Build history of the part. All positions in model axes, mm. Give positions to 0.01 mm unless a question says otherwise; leave off trailing zeros. One line per item, written item: value. Start each with the question number.
from build123d import *

# Parameters (mm, degrees)
BOSS_EXTRUDE1_DEPTH   = 1000
SKETCH3_R             = 3.4
CUT_EXTRUDE1_DEPTH    = 1000
CUT_EXTRUDE2_DEPTH    = 1000
FILLET1_R             = 1
FILLET2_R             = 1
FILLET3_R             = 1
CUT_EXTRUDE3_DEPTH    = 1000
CUT_EXTRUDE4_DEPTH    = 1000
FILLET4_R             = 1
FILLET5_R             = 1
FILLET6_R             = 1
FILLET7_R             = 1
FILLET8_R             = 1
FILLET9_R             = 1
FILLET10_R            = 1
FILLET11_R            = 1
MIRROR11_COPY_1_DEPTH = 1000
MIRROR11_COPY_2_DEPTH = 1000
CUT_EXTRUDE5_DEPTH    = 1000


with BuildPart() as part:
    # Sketch1 → Boss-Extrude1 (new body)
    with BuildSketch(Plane(origin=(0, 0, 0), x_dir=(1, 0, 0), z_dir=(0, 1, 0))):
        with BuildLine():
            Line((5, 0), (75, 0))
            ThreePointArc((75, 0), (78.535533906, -1.464466094), (80, -5))
            Line((80, -5), (80, -35))
            ThreePointArc((80, -35), (78.535533906, -38.535533906), (75, -40))
            Line((75, -40), (5, -40))
            ThreePointArc((5, -40), (1.464466094, -38.535533906), (0, -35))
            Line((0, -35), (0, -5))
            ThreePointArc((0, -5), (1.464466094, -1.464466094), (5, 0))
        make_face()
    extrude(amount=BOSS_EXTRUDE1_DEPTH)

    # Sketch3 → Cut-Extrude1 (cut)
    with BuildSketch(Plane(origin=(0, 1000, 0), x_dir=(1, 0, 0), z_dir=(0, 1, 0))):
        with Locations(Location((20, -20, 0), (0, 0, 270))):
            Circle(SKETCH3_R)
    cut_extrude1 = extrude(amount=-CUT_EXTRUDE1_DEPTH, mode=Mode.SUBTRACT)

    # Mirror3: Cut-Extrude1 across plane
    add(cut_extrude1.mirror(Plane(origin=(40, 0, 0), x_dir=(0, 0, 1), z_dir=(1, 0, 0))), mode=Mode.SUBTRACT)

    # Sketch7 → Cut-Extrude2 (cut)
    with BuildSketch(Plane(origin=(0, 0, 0), x_dir=(-1, 0, 0), z_dir=(0, -1, 0))):
        with BuildLine():
            Line((-15.9, -40), (-24.1, -40))
            Line((-24.1, -40), (-24.1, -36.5))
            ThreePointArc((-24.1, -36.5), (-24.392893219, -35.792893219), (-25.1, -35.5))
            Line((-25.1, -35.5), (-29.489753594, -35.5))
            ThreePointArc((-29.489753594, -35.5), (-30.415270825, -34.8787055), (-30.190750526, -33.786835712))
            Line((-30.190750526, -33.786835712), (-24.391814382, -28.086835712))
            ThreePointArc((-24.391814382, -28.086835712), (-24.069522951, -27.874482769), (-23.69081745, -27.8))
            Line((-23.69081745, -27.8), (-16.309186536, -27.8))
            ThreePointArc((-16.309186536, -27.8), (-15.930477876, -27.874484063), (-15.608184734, -28.086840499))
            Line((-15.608184734, -28.086840499), (-9.809327805, -33.786840499))
            ThreePointArc((-9.809327805, -33.786840499), (-9.584813669, -34.87870866), (-10.510329607, -35.5))
            Line((-10.510329607, -35.5), (-14.9, -35.5))
            ThreePointArc((-14.9, -35.5), (-15.607106781, -35.792893219), (-15.9, -36.5))
            Line((-15.9, -36.5), (-15.9, -40))
        make_face()
    cut_extrude2 = extrude(amount=-CUT_EXTRUDE2_DEPTH, mode=Mode.SUBTRACT)

    # Fillet1
    fillet1_edges = [part.edges().sort_by_distance(p)[0] for p in [
        (15.9, 500, 40),
        (24.1, 500, 40),
    ]]
    fillet(fillet1_edges, radius=FILLET1_R)

    # Mirror8: Cut-Extrude2 across plane
    add(cut_extrude2.mirror(Plane(origin=(40, 0, 0), x_dir=(0, 0, 1), z_dir=(1, 0, 0))), mode=Mode.SUBTRACT)

    # Fillet2
    fillet2_edges = [part.edges().sort_by_distance(p)[0] for p in [
        (55.9, 500, 40),
    ]]
    fillet(fillet2_edges, radius=FILLET2_R)

    # Fillet3
    fillet3_edges = [part.edges().sort_by_distance(p)[0] for p in [
        (64.1, 500, 40),
    ]]
    fillet(fillet3_edges, radius=FILLET3_R)

    # Sketch9 → Cut-Extrude3 (cut)
    with BuildSketch(Plane(origin=(0, 0, 0), x_dir=(1, 0, 0), z_dir=(0, 1, 0))):
        with BuildLine():
            Line((14.899846923, -4.500713815), (10.450461284, -4.500713815))
            ThreePointArc((10.450461284, -4.500713815), (9.526581751, -5.118030383), (9.743354502, -6.207820596))
            Line((9.743354502, -6.207820596), (15.442640687, -11.907106781))
            ThreePointArc((15.442640687, -11.907106781), (15.767064036, -12.123879533), (16.149747468, -12.2))
            Line((16.149747468, -12.2), (23.850252532, -12.2))
            ThreePointArc((23.850252532, -12.2), (24.232935964, -12.123879533), (24.557359313, -11.907106781))
            Line((24.557359313, -11.907106781), (30.257359313, -6.207106781))
            ThreePointArc((30.257359313, -6.207106781), (30.474132064, -5.117316568), (29.550252532, -4.5))
            Line((29.550252532, -4.5), (25.099846964, -4.5))
            ThreePointArc((25.099846964, -4.5), (24.392724723, -4.207091321), (24.099846965, -3.499956273))
            Line((24.099846965, -3.499956273), (24.100000008, 0))
            Line((24.100000008, 0), (15.9, 0))
            Line((15.9, 0), (15.899846922, -3.500757542))
            ThreePointArc((15.899846922, -3.500757542), (15.606938244, -4.207836056), (14.899846923, -4.500713815))
        make_face()
    cut_extrude3 = extrude(amount=CUT_EXTRUDE3_DEPTH, mode=Mode.SUBTRACT)

    # Mirror9: Cut-Extrude3 across plane
    add(cut_extrude3.mirror(Plane(origin=(40, 0, 0), x_dir=(0, 0, 1), z_dir=(1, 0, 0))), mode=Mode.SUBTRACT)

    # Sketch10 → Cut-Extrude4 (cut)
    with BuildSketch(Plane(origin=(0, 0, 0), x_dir=(1, 0, 0), z_dir=(0, 1, 0))):
        with BuildLine():
            Line((4.5, -14.9), (4.5, -10.58605332))
            ThreePointArc((4.5, -10.58605332), (5.126159695, -9.658560233), (6.220486853, -9.892584724))
            Line((6.220486853, -9.892584724), (11.920486853, -15.814662646))
            ThreePointArc((11.920486853, -15.814662646), (12.127493087, -16.134290938), (12.2, -16.508131242))
            Line((12.2, -16.508131242), (12.2, -23.491868758))
            ThreePointArc((12.2, -23.491868758), (12.127493087, -23.865709062), (11.920486853, -24.185337354))
            Line((11.920486853, -24.185337354), (6.220486853, -30.107415276))
            ThreePointArc((6.220486853, -30.107415276), (5.126159695, -30.341439767), (4.5, -29.41394668))
            Line((4.5, -29.41394668), (4.5, -25.1))
            ThreePointArc((4.5, -25.1), (4.207106781, -24.392893219), (3.5, -24.1))
            Line((3.5, -24.1), (0, -24.1))
            Line((0, -24.1), (0, -15.9))
            Line((0, -15.9), (3.5, -15.9))
            ThreePointArc((3.5, -15.9), (4.207106781, -15.607106781), (4.5, -14.9))
        make_face()
    cut_extrude4 = extrude(amount=CUT_EXTRUDE4_DEPTH, mode=Mode.SUBTRACT)

    # Fillet4
    fillet4_edges = [part.edges().sort_by_distance(p)[0] for p in [
        (24.100000008, 500, 0),
    ]]
    fillet(fillet4_edges, radius=FILLET4_R)

    # Fillet5
    fillet5_edges = [part.edges().sort_by_distance(p)[0] for p in [
        (64.1, 500, 0),
    ]]
    fillet(fillet5_edges, radius=FILLET5_R)

    # Fillet6
    fillet6_edges = [part.edges().sort_by_distance(p)[0] for p in [
        (55.899999992, 500, 0),
    ]]
    fillet(fillet6_edges, radius=FILLET6_R)

    # Fillet7
    fillet7_edges = [part.edges().sort_by_distance(p)[0] for p in [
        (15.9, 500, 0),
    ]]
    fillet(fillet7_edges, radius=FILLET7_R)

    # Fillet8
    fillet8_edges = [part.edges().sort_by_distance(p)[0] for p in [
        (0, 500, 24.1),
    ]]
    fillet(fillet8_edges, radius=FILLET8_R)

    # Fillet9
    fillet9_edges = [part.edges().sort_by_distance(p)[0] for p in [
        (0, 500, 15.9),
    ]]
    fillet(fillet9_edges, radius=FILLET9_R)

    # Mirror10: Cut-Extrude4 across plane
    add(cut_extrude4.mirror(Plane(origin=(40, 0, 0), x_dir=(0, 0, 1), z_dir=(1, 0, 0))), mode=Mode.SUBTRACT)

    # Fillet10
    fillet10_edges = [part.edges().sort_by_distance(p)[0] for p in [
        (80, 500, 15.9),
    ]]
    fillet(fillet10_edges, radius=FILLET10_R)

    # Fillet11
    fillet11_edges = [part.edges().sort_by_distance(p)[0] for p in [
        (80, 500, 24.1),
    ]]
    fillet(fillet11_edges, radius=FILLET11_R)

    # Mirror11 copy 1 sketch → Mirror11 copy 1 (cut)
    with BuildSketch(Plane(origin=(40, 0, 0), x_dir=(1, 0, 0), z_dir=(0, 1, 0))):
        with BuildLine():
            Line((4.5, -14.9), (4.5, -10.58605332))
            ThreePointArc((4.5, -10.58605332), (5.126159695, -9.658560233), (6.220486853, -9.892584724))
            Line((6.220486853, -9.892584724), (11.920486853, -15.814662646))
            ThreePointArc((11.920486853, -15.814662646), (12.127493087, -16.134290938), (12.2, -16.508131242))
            Line((12.2, -16.508131242), (12.2, -23.491868758))
            ThreePointArc((12.2, -23.491868758), (12.127493087, -23.865709062), (11.920486853, -24.185337354))
            Line((11.920486853, -24.185337354), (6.220486853, -30.107415276))
            ThreePointArc((6.220486853, -30.107415276), (5.126159695, -30.341439767), (4.5, -29.41394668))
            Line((4.5, -29.41394668), (4.5, -25.1))
            ThreePointArc((4.5, -25.1), (4.207106781, -24.392893219), (3.5, -24.1))
            Line((3.5, -24.1), (0, -24.1))
            Line((0, -24.1), (0, -15.9))
            Line((0, -15.9), (3.5, -15.9))
            ThreePointArc((3.5, -15.9), (4.207106781, -15.607106781), (4.5, -14.9))
        make_face()
    extrude(amount=MIRROR11_COPY_1_DEPTH, mode=Mode.SUBTRACT)

    # Mirror11 copy 2 sketch → Mirror11 copy 2 (cut)
    with BuildSketch(Plane(origin=(120, 0, 0), x_dir=(-1, 0, 0), z_dir=(0, 1, 0))):
        with BuildLine():
            Line((4.5, 14.9), (4.5, 10.58605332))
            ThreePointArc((4.5, 10.58605332), (5.126159695, 9.658560233), (6.220486853, 9.892584724))
            Line((6.220486853, 9.892584724), (11.920486853, 15.814662646))
            ThreePointArc((11.920486853, 15.814662646), (12.127493087, 16.134290938), (12.2, 16.508131242))
            Line((12.2, 16.508131242), (12.2, 23.491868758))
            ThreePointArc((12.2, 23.491868758), (12.127493087, 23.865709062), (11.920486853, 24.185337354))
            Line((11.920486853, 24.185337354), (6.220486853, 30.107415276))
            ThreePointArc((6.220486853, 30.107415276), (5.126159695, 30.341439767), (4.5, 29.41394668))
            Line((4.5, 29.41394668), (4.5, 25.1))
            ThreePointArc((4.5, 25.1), (4.207106781, 24.392893219), (3.5, 24.1))
            Line((3.5, 24.1), (0, 24.1))
            Line((0, 24.1), (0, 15.9))
            Line((0, 15.9), (3.5, 15.9))
            ThreePointArc((3.5, 15.9), (4.207106781, 15.607106781), (4.5, 14.9))
        make_face()
    extrude(amount=MIRROR11_COPY_2_DEPTH, mode=Mode.SUBTRACT)

    # Mirror12: Cut-Extrude4 across plane
    add(cut_extrude4.mirror(Plane.ZY.offset(-20)), mode=Mode.SUBTRACT)

    # Sketch12 → Cut-Extrude5 (cut)
    with BuildSketch(Plane(origin=(0, 0, 0), x_dir=(-1, 0, 0), z_dir=(0, -1, 0))):
        with BuildLine():
            Line((-28.079513147, -24.185337354), (-39.327067998, -35.871108628))
            ThreePointArc((-39.327067998, -35.871108628), (-40.049082116, -36.177638866), (-40.770156561, -35.868904648))
            Line((-40.770156561, -35.868904648), (-51.922601709, -24.210885791))
            ThreePointArc((-51.922601709, -24.210885791), (-52.128062958, -23.892044517), (-52.2, -23.519621175))
            Line((-52.2, -23.519621175), (-52.2, -16.508131242))
            ThreePointArc((-52.2, -16.508131242), (-52.127493087, -16.134290938), (-51.920486853, -15.814662646))
            Line((-51.920486853, -15.814662646), (-40.720486853, -4.17829901))
            ThreePointArc((-40.720486853, -4.17829901), (-40, -3.871767606), (-39.279513147, -4.17829901))
            Line((-39.279513147, -4.17829901), (-28.079513147, -15.814662646))
            ThreePointArc((-28.079513147, -15.814662646), (-27.872506913, -16.134290938), (-27.8, -16.508131242))
            Line((-27.8, -16.508131242), (-27.8, -23.491868758))
            ThreePointArc((-27.8, -23.491868758), (-27.872506913, -23.865709062), (-28.079513147, -24.185337354))
        make_face()
    extrude(amount=-CUT_EXTRUDE5_DEPTH, mode=Mode.SUBTRACT)


solid = part.part
1) Drill centre lines: line 1 (X direction, y = 456.5, z = 20); line 2 (Z direction, x = 59.5, y = 647.5); line 3 (Z direction, x = 41, y = 666). Where is each one in solid material? Low to high.
2) Slice it at A-A (y = 852.5). State how many separate pieces and enclosed holes the cut face has, plus the area to 3 significant figures.
3) Drop flat-ended pins along their axis: P1, Ø2, axis at y = 449, z = 37.5, coming from the -X side; P2, Ø1.2, axis at y = 591.5, z = 38, coming from the +X side; P3, Ø1.2, axis at x = 2.5, y = 272, coming from the +Z side. Give the stop position or say it passes through.
Results list:
1. line 1: x = 12.2 to 16.6, 23.4 to 27.8, 52.2 to 56.6, 63.4 to 67.8
1. line 2: z = 12.2 to 16.64, 23.36 to 27.8
1. line 3: z = 0 to 4.47, 35.63 to 40
2. separate pieces: 1
2. enclosed holes: 3
2. area: 1,660 mm²
3. P1: stops at x = 0.23
3. P2: stops at x = 79.39
3. P3: stops at z = 39.62
